The listing builds one solid part. Answer for the finished solid, in the listing's coordinates (mm). A direction names the side the tool comes from. Give positions to 0.01 mm unless a question says otherwise; leave off trailing zeros. Write each loop counter-clockwise with the first axis right and the second up, starting at its lowest first coordinate (ties: lowest second). Pieces come first, ordered by that corner, then holes. Notation, with made-up numbers: M 3.25,36 L 14.25,36 A21 ccw 14.25,67 Z; hole C 9,18.25 d11. An arc over 180 degrees is marked long. Return JSON: item names as keys, results as strings.
from build123d import *

# Parameters (mm, degrees)
SKETCH1_R               = 4.953
BOSS_EXTRUDE1_DEPTH     = 21.336
BOSS_EXTRUDE2_START     = -10.414
SKETCH2_R               = 6.858
BOSS_EXTRUDE2_DEPTH     = 2.54
CUT_EXTRUDE1_DEPTH      = 24.436920105
CUT_EXTRUDE1_DEPTH_BACK = 24.436920105
SKETCH3_W               = 1.27
SKETCH3_H               = 2.794
CUT_EXTRUDE2_DEPTH      = 24.436920105
CUT_EXTRUDE2_DEPTH_BACK = 24.436920105
SKETCH4_W               = 1.27
SKETCH4_H               = 2.794


with BuildPart() as part:
    # Sketch1 → Boss-Extrude1 (new body)
    with BuildSketch(Plane.XY):
        Circle(SKETCH1_R)
    extrude(amount=BOSS_EXTRUDE1_DEPTH)

    # Sketch2 → Boss-Extrude2 (add)
    with BuildSketch(Plane.XY.offset(21.336).offset(BOSS_EXTRUDE2_START)):
        Circle(SKETCH2_R)
    extrude(amount=-BOSS_EXTRUDE2_DEPTH)

    # Sketch3 → Cut-Extrude1 (cut, two sides: drawn at the far end of the back side and taken through both)
    with BuildSketch(Plane(origin=(0, 0, 0), x_dir=(1, 0, 0), z_dir=(0, 1, 0)).offset(-CUT_EXTRUDE1_DEPTH_BACK)):
        with Locations((4.318, -2.667)):
            Rectangle(SKETCH3_W, SKETCH3_H)
        with Locations((-4.318, -2.667)):
            Rectangle(SKETCH3_W, SKETCH3_H)
    extrude(amount=CUT_EXTRUDE1_DEPTH + CUT_EXTRUDE1_DEPTH_BACK, mode=Mode.SUBTRACT)

    # Sketch4 → Cut-Extrude2 (cut, two sides: drawn at the far end of the back side and taken through both)
    with BuildSketch(Plane(origin=(0, 0, 0), x_dir=(1, 0, 0), z_dir=(0, 1, 0)).offset(-CUT_EXTRUDE2_DEPTH_BACK)):
        with Locations((4.318, -18.669)):
            Rectangle(SKETCH4_W, SKETCH4_H)
        with Locations((-4.318, -18.669)):
            Rectangle(SKETCH4_W, SKETCH4_H)
    extrude(amount=CUT_EXTRUDE2_DEPTH + CUT_EXTRUDE2_DEPTH_BACK, mode=Mode.SUBTRACT)


solid = part.part
Item 1: A cutting plane is placed at D-D, the plane z = 6.5. Write down the section's boundary in (x, y).
Geometry results:
{"outline": "C 0,0 d9.91"}
Item 2: Which of the six approach directions +Z, -Z, +X, -X, +Y, -Y give full straight-line access (tool end or side, diameter ignored) to faces 1 (the cylindrical face through (-0.64, 4.91, 16.06)), 2 (the flat face through (4, 0, 17.272)), 3 (the flat face through (-3.683, 0, 19)), 4 (the cylindrical face through (-0.64, 4.91, 4.13)), 5 (the cylindrical face through (-1.487, -6.695, 9.67))?
Geometry results:
{"face 1": "+Z", "face 2": "+X, +Y, -Y", "face 3": "-X, +Y, -Y", "face 4": "-Z", "face 5": "+Z, -Z"}
Item 3: Given pin 1 Ø3 at (y, z) = (2.5, 4.5) entering from -X; pin 2 Ø0.8 at (y, z) = (-1, 19) entering from -X; pin 3 Ø2 at (y, z) = (-1.5, 2) entering from +X, each flat-ended and moving along its own axis, determine where each tip first touches the part or whether it passes through.
Geometry results:
{"pin 1": "stops at x = -4.85", "pin 2": "stops at x = -3.68", "pin 3": "stops at x = 4.89"}
Item 4: Find the intervals of material crossed by line 1 (X direction, y = -0.25, z = 2.75); line 2 (Z direction, x = -5.5, y = 2.75); line 3 (X direction, y = -0.25, z = 10.25), in increasing order.
Geometry results:
{"line 1": "x = -3.68 to 3.68", "line 2": "z = 8.38 to 10.92", "line 3": "x = -6.85 to 6.85"}
Item 5: A cutting plane is placed at B-B, the plane x = 4.25. Write down the section's boundary in (y, z).
Geometry results:
{"outline": "M -5.38,8.38 L -2.54,8.38 L -2.54,4.06 L 2.54,4.06 L 2.54,8.38 L 5.38,8.38 L 5.38,10.92 L 2.54,10.92 L 2.54,17.27 L -2.54,17.27 L -2.54,10.92 L -5.38,10.92 Z; M -2.54,0 L 2.54,0 L 2.54,1.27 L -2.54,1.27 Z; M -2.54,20.07 L 2.54,20.07 L 2.54,21.34 L -2.54,21.34 Z"}
Item 6: Determine the mould class of faces 6 (the flat face through (-4, 0, 1.27)), 7 (the flat face through (4, 0, 4.064)), 8 (the flat face through (2, -5, 8.382)), 9 (the flat face through (0, 0, 21.336)) for opening direction Z: +Z half, -Z half, draft (parallel to the pull), parting line (faces both ways), or undercut.
Geometry results:
{"face 6": "undercut", "face 7": "undercut", "face 8": "-Z half", "face 9": "+Z half"}
Item 7: A cutting plane is placed at A-A, the plane y = 0. Write down the section's boundary in (x, z).
Geometry results:
{"outline": "M -6.86,8.38 L -4.95,8.38 L -4.95,4.06 L -3.68,4.06 L -3.68,1.27 L -4.95,1.27 L -4.95,0 L 4.95,0 L 4.95,1.27 L 3.68,1.27 L 3.68,4.06 L 4.95,4.06 L 4.95,8.38 L 6.86,8.38 L 6.86,10.92 L 4.95,10.92 L 4.95,17.27 L 3.68,17.27 L 3.68,20.07 L 4.95,20.07 L 4.95,21.34 L -4.95,21.34 L -4.95,20.07 L -3.68,20.07 L -3.68,17.27 L -4.95,17.27 L -4.95,10.92 L -6.86,10.92 Z"}
Item 8: A cutting plane is placed at C-C, the plane x = 0. Write down the section's boundary in (y, z).
Geometry results:
{"outline": "M -6.86,8.38 L -4.95,8.38 L -4.95,0 L 4.95,0 L 4.95,8.38 L 6.86,8.38 L 6.86,10.92 L 4.95,10.92 L 4.95,21.34 L -4.95,21.34 L -4.95,10.92 L -6.86,10.92 Z"}
